Read the model definition and answer for the solid it produces. Units are mm, in the model's axes. Face numbers are marked on the shaded views. A direction names the side the tool comes from. Round coordinates to 2 decimals unless told otherwise and drop trailing zeros. Order: outer loops, then holes, each group sorted by start corner. A loop starts at its lowest first (then second) coordinate and runs counter-clockwise, first axis right, second up. Notation, with made-up numbers: M 31.5,-16.5 L 90.5,-16.5 A26 cw 90.5,6.5 Z; hole C 0.25,-2 d10. An arc over 180 degrees is marked long. Answer as CSV lines item,"result".
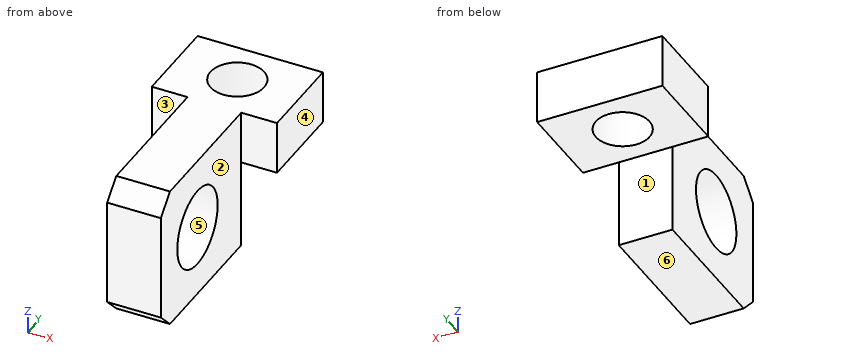
```python
from build123d import *

# Parameters (mm, degrees)
SKETCH7_R          = 1.905
BASE_DEPTH         = 10.16
LEVER_HOLE_REACH   = 23.199
SKETCH8_R          = 2.794
CHAMFER2_SIZE      = 1.27
SKETCH9_W          = 8.89
SKETCH9_H          = 6.35
CUT_EXTRUDE4_DEPTH = 6.35


with BuildPart() as part:
    # Sketch7 → base (new body)
    with BuildSketch(Plane(origin=(0, 0, 0), x_dir=(0, 1, 0), z_dir=(0, 0, 1))):
        Polygon((11.138733525, 0), (11.138733525, -2.54), (17.488733525, -2.54), (17.488733525, 6.35), (11.138733525, 6.35), (11.138733525, 3.81), (0, 3.81), (0, 0), align=None)
        with Locations(Location((14.313733525, 1.905, 0), (0, 0, 270))):
            Circle(SKETCH7_R, mode=Mode.SUBTRACT)
    extrude(amount=BASE_DEPTH)

    # Sketch8 → lever_hole (cut, up to next)
    with BuildSketch(Plane.YZ, mode=Mode.PRIVATE) as lever_hole_sk1:
        with Locations(Location((5.08, 5.08, 0), (0, 0, 270))):
            Circle(SKETCH8_R)
    lever_hole_tool1 = extrude(lever_hole_sk1.sketch, amount=-LEVER_HOLE_REACH, mode=Mode.PRIVATE) & part.part
    add(lever_hole_tool1.solids().sort_by_distance((0, 5.08, 5.08))[0], mode=Mode.SUBTRACT)

    # Chamfer2
    chamfer2_edges = [part.edges().sort_by_distance(p)[0] for p in [
        (-1.905, 0, 0),
        (-1.905, 0, 10.16),
    ]]
    chamfer(chamfer2_edges, length=CHAMFER2_SIZE)

    # Sketch9 → Cut-Extrude4 (cut)
    with BuildSketch(Plane(origin=(0, 0, 0), x_dir=(1, 0, 0), z_dir=(0, 0, -1))):
        with Locations((-1.905, -14.313733525)):
            Rectangle(SKETCH9_W, SKETCH9_H)
    extrude(amount=-CUT_EXTRUDE4_DEPTH, mode=Mode.SUBTRACT)


solid = part.part
```
Item 1: A cutting plane is placed at D-D, the plane z = 5.5. Determine the outline of the cut face in (x, y), and give its area (3 significant figures).
Ans:
outline,"M -3.81,0 L 0,0 L 0,2.32 L -3.81,2.32 Z; M -3.81,7.84 L 0,7.84 L 0,11.14 L -3.81,11.14 Z"
area,"21.4 mm2"
Item 2: Find the intervals of material crossed by probe 1 along Z at (x, y) = (-2.5, 5); probe 2 along Y at (x, z) = (-1.3, 5.08); probe 3 along Y at (x, z) = (-3.25, 7.5), in increasing order. Write a range as [from, to].
Ans:
probe 1,"[0, 2.29], [7.87, 10.16]"
probe 2,"[0, 2.29], [7.87, 11.14]"
probe 3,"[0, 3.68], [6.48, 12.96], [15.66, 17.49]"
Item 3: Determine the mould class of the marked faces 4, 5 and 6 for opening direction Z: +Z half, -Z half, draft (parallel to the pull), parting line (faces both ways), or undercut.
Ans:
face 4,"draft"
face 5,"undercut"
face 6,"-Z half"
Item 4: A cutting plane is placed at B-B, the plane z = 6.75. Determine the outline of the cut face in (x, y) (3 decimals), and give its area (3 significant figures).
Ans:
outline,"M -6.35,11.139 L -3.81,11.139 L -3.81,7.32 L 0,7.32 L 0,11.139 L 2.54,11.139 L 2.54,17.489 L -6.35,17.489 Z; M -3.81,0 L 0,0 L 0,2.84 L -3.81,2.84 Z; hole C -1.905,14.314 d3.81"
area,"70.4 mm2"
Item 5: Flat-ended cylindrical pins translate along their axes: pin 1 (5 mm diameter, centred on y = 6.5, z = 7, fed in from -X); pin 2 (1.9 mm diameter, centred on x = -2.5, y = 13, fed in from -Z); pin 3 (1 mm diameter, centred on y = 6.5, z = 2.5, fed in from +X). Find the tip coordinate at first contact, or state that the pin passes through.
Ans:
pin 1,"x = -3.81"
pin 2,"z = 6.35"
pin 3,"x = 0"
Item 6: A tool of negligible diameter and unlimited length cuts with its end or side. For the marked faces 1, 2 and 3, from which of +Z, -Z, +X, -X, +Y, -Y can it reach the whole face along a straight path? Write none if from no direction.
Ans:
face 1,"-Z, +X, -X, +Y"
face 2,"+Z, -Z, +X, -Y"
face 3,"+Z, -Z, -X, -Y"
Item 7: A cutting plane is placed at C-C, the plane x = -3.5. Determine the outline of the cut face in (y, z).
Ans:
outline,"M 0,1.27 L 1.27,0 L 11.14,0 L 11.14,6.35 L 13.27,6.35 L 13.27,10.16 L 1.27,10.16 L 0,8.89 Z; M 15.36,6.35 L 17.49,6.35 L 17.49,10.16 L 15.36,10.16 Z; hole C 5.08,5.08 d5.59"
Item 8: A cutting plane is placed at A-A, the plane y = 5.08. Determine the outline of the cut face in (x, z).
Ans:
outline,"M -3.81,0 L 0,0 L 0,2.29 L -3.81,2.29 Z; M -3.81,7.87 L 0,7.87 L 0,10.16 L -3.81,10.16 Z"
